Part model, mm, in its own coordinate system. Round coordinates to 2 decimals unless told otherwise and drop trailing zeros. Write each loop counter-clockwise with the first axis right and the second up, starting at its lowest first coordinate (ties: lowest second). Pieces come first, ordered by that corner, then holes. Notation, with made-up numbers: M -12,-20 L 9,-20 A34 cw 9,13 Z; hole C 55.25,62.5 d10. An arc over 180 degrees is marked long. Use a Markdown table: item, result. Add a question column.
1) Slice it at B-B on z = -36.5. Write the cut outline in (x, y), plus the area to 3 significant figures.
2) Slice it at A-A on x = -40. Write the cut outline in (y, z), plus the area to 3 significant figures.
3) Slice it at C-C on y = 1.75. Write the cut outline in (x, z).
4) Wall check: probe 1 along X at (y, z) = (4.25, -37); probe 2 along Z at (x, y) = (53.5, 5.25). Give the ranges that are in metal, low to high.
```python
from build123d import *

# Parameters (mm, degrees)
SKETCH1_W           = 150
SKETCH1_H           = 150
SKETCH1_W_2         = 20
SKETCH1_H_2         = 10
BOSS_EXTRUDE1_DEPTH = 10


with BuildPart() as part:
    # Sketch1 → Boss-Extrude1 (new body)
    with BuildSketch(Plane(origin=(0, 0, 0), x_dir=(1, 0, 0), z_dir=(0, 1, 0))):
        Rectangle(SKETCH1_W, SKETCH1_H)
        with Locations((-45, 35)):
            Rectangle(SKETCH1_W_2, SKETCH1_H_2, mode=Mode.SUBTRACT)
        with Locations((0, 35)):
            Rectangle(SKETCH1_W_2, SKETCH1_H_2, mode=Mode.SUBTRACT)
        with Locations((45, 35)):
            Rectangle(SKETCH1_W_2, SKETCH1_H_2, mode=Mode.SUBTRACT)
    extrude(amount=BOSS_EXTRUDE1_DEPTH)


solid = part.part
```
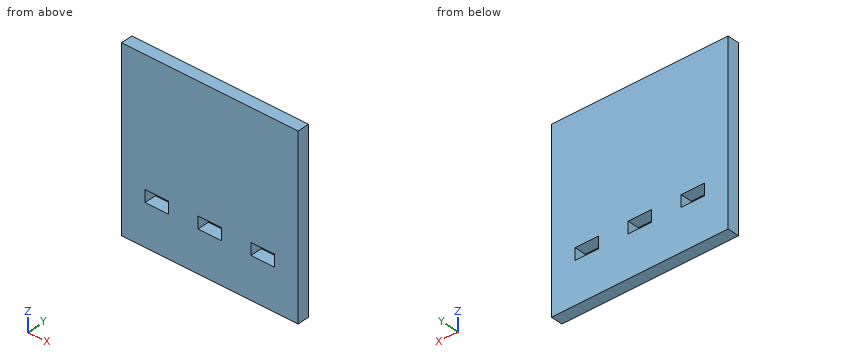
Entries:
| question | item | result |
|---|---|---|
| 1 | outline | M -75,0 L -55,0 L -55,10 L -75,10 Z; M -35,0 L -10,0 L -10,10 L -35,10 Z; M 10,0 L 35,0 L 35,10 L 10,10 Z; M 55,0 L 75,0 L 75,10 L 55,10 Z |
| 1 | area | 900 mm^2 |
| 2 | outline | M 0,-75 L 10,-75 L 10,-40 L 0,-40 Z; M 0,-30 L 10,-30 L 10,75 L 0,75 Z |
| 2 | area | 1,400 mm^2 |
| 3 | outline | M -75,-75 L 75,-75 L 75,75 L -75,75 Z; hole M -55,-40 L -35,-40 L -35,-30 L -55,-30 Z; hole M -10,-40 L 10,-40 L 10,-30 L -10,-30 Z; hole M 35,-40 L 55,-40 L 55,-30 L 35,-30 Z |
| 4 | probe 1 | x = -75 to -55, -35 to -10, 10 to 35, 55 to 75 |
| 4 | probe 2 | z = -75 to -40, -30 to 75 |
